```python
from build123d import *

# Parameters (mm, degrees)
F0_W           = 15.6
F0_H           = 5.8
F1_DEPTH       = 13.4
F2_W           = 1.5
F2_H           = 6.25
F3_DEPTH       = 1
F4_W           = 1.5
F4_H           = 6.25
F5_DEPTH       = 1
F6_W           = 13.6
F6_H           = 1
F7_DEPTH       = 1
F8_W           = 1.5
F8_H           = 6.3
F9_DEPTH       = 1
F10_W          = 1.3
F10_H          = 1.3
F11_DEPTH      = 13.401
F12_W          = 3.1
F12_H          = 4.1
F12_W_2        = 1.3
F12_H_2        = 1.3
F13_DEPTH      = 12.9
F15_DEPTH      = 3.75
F15_DEPTH_BACK = 3.75
F16_W          = 2.5
F16_H          = 8.7
F17_DEPTH      = 0.5


with BuildPart() as f1:
    # F0 (on Top) → F1 (new body)
    with BuildSketch(Plane.XY):
        Rectangle(F0_W, F0_H)
    extrude(amount=F1_DEPTH)

    # F2 (on face) → F3 (join)
    with BuildSketch(Plane.YZ.offset(7.8)):
        with Locations((3.65, 3.125)):
            Rectangle(F2_W, F2_H)
    extrude(amount=-F3_DEPTH)

    # F4 (on face) → F5 (join)
    with BuildSketch(Plane(origin=(-7.8, 0, 0), x_dir=(0, -1, 0), z_dir=(-1, 0, 0))):
        with Locations((-3.65, 3.125)):
            Rectangle(F4_W, F4_H)
    extrude(amount=-F5_DEPTH)

    # F6 (on face) → F7 (join)
    with BuildSketch(Plane.XZ.offset(2.9)):
        with Locations((0, 12.9)):
            Rectangle(F6_W, F6_H)
    extrude(amount=F7_DEPTH)

    # F8 (on face) → F9 (cut)
    with BuildSketch(Plane.XZ.offset(2.9)):
        with Locations((-6, 3.15)):
            Rectangle(F8_W, F8_H)
        with Locations((-2, 3.15)):
            Rectangle(F8_W, F8_H)
        with Locations((2, 3.15)):
            Rectangle(F8_W, F8_H)
        with Locations((6, 3.15)):
            Rectangle(F8_W, F8_H)
    extrude(amount=-F9_DEPTH, mode=Mode.SUBTRACT)

    # F10 (on Top) → F11 (cut, through all)
    with BuildSketch(Plane.XY):
        with Locations((5.94, 0.95)):
            Rectangle(F10_W, F10_H)
        with Locations((1.98, 0.95)):
            Rectangle(F10_W, F10_H)
        with Locations((-1.98, 0.95)):
            Rectangle(F10_W, F10_H)
        with Locations((-5.94, 0.95)):
            Rectangle(F10_W, F10_H)
    extrude(amount=F11_DEPTH, mode=Mode.SUBTRACT)

    # F12 (on face) → F13 (cut)
    with BuildSketch(Plane.XY.offset(13.4)):
        with Locations((-5.94, 0.1)):
            Rectangle(F12_W, F12_H)
        with Locations((-5.94, 0.95)):
            Rectangle(F12_W_2, F12_H_2, mode=Mode.SUBTRACT)
        with Locations((-1.98, 0.1)):
            Rectangle(F12_W, F12_H)
        with Locations((-1.98, 0.95)):
            Rectangle(F12_W_2, F12_H_2, mode=Mode.SUBTRACT)
        with Locations((1.98, 0.1)):
            Rectangle(F12_W, F12_H)
        with Locations((1.98, 0.95)):
            Rectangle(F12_W_2, F12_H_2, mode=Mode.SUBTRACT)
        with Locations((5.94, 0.1)):
            Rectangle(F12_W, F12_H)
        with Locations((5.94, 0.95)):
            Rectangle(F12_W_2, F12_H_2, mode=Mode.SUBTRACT)
    extrude(amount=-F13_DEPTH, mode=Mode.SUBTRACT)

    # F14 (on Right) → F15 (join, two sides)
    with BuildSketch(Plane.YZ) as f15_sk:
        with BuildLine():
            Line((3.5, 13.4), (2.9, 13.4))
            Line((2.9, 13.4), (2.9, 5.7))
            Line((2.9, 5.7), (3.5, 5.7))
            Line((3.5, 5.7), (3.5, 5.91))
            ThreePointArc((3.5, 5.91), (3.672807, 6.327193), (4.09, 6.5))
            Line((4.09, 6.5), (4.11, 6.5))
            ThreePointArc((4.11, 6.5), (4.527193, 6.327193), (4.7, 5.91))
            Line((4.7, 5.91), (4.7, 2.3))
            Line((4.7, 2.3), (6.1, 2.3))
            Line((6.1, 2.3), (6.1, 11))
            Line((6.1, 11), (7.132015, 11))
            Line((7.132015, 11), (7.132015, 12))
            Line((7.132015, 12), (4.7, 12))
            Line((4.7, 12), (4.7, 8.09))
            ThreePointArc((4.7, 8.09), (4.527193, 7.672807), (4.11, 7.5))
            Line((4.11, 7.5), (4.09, 7.5))
            ThreePointArc((4.09, 7.5), (3.672807, 7.672807), (3.5, 8.09))
            Line((3.5, 8.09), (3.5, 13.4))
        make_face()
    extrude(amount=F15_DEPTH)
    extrude(f15_sk.sketch, amount=-F15_DEPTH_BACK)

    # F16 (on face) → F17 (cut)
    with BuildSketch(Plane(origin=(0, 6.1, 0), x_dir=(-1, 0, 0), z_dir=(0, 1, 0))):
        with Locations((-2.5, 6.65)):
            Rectangle(F16_W, F16_H)
        with Locations((2.5, 6.65)):
            Rectangle(F16_W, F16_H)
    extrude(amount=-F17_DEPTH, mode=Mode.SUBTRACT)


solid = f1.part
```
Check sheet for the modelled part. Datum: model origin and axes. Units: mm. A direction names the side the tool comes from. Round coordinates to 2 decimals unless told otherwise and drop trailing zeros. Loops run counter-clockwise (first coordinate to the right, second up) from the corner with the lowest first, then second, coordinate; pieces in that order, holes last. Notation, with made-up numbers: (25.25, -13.5) -> (71.25, -13.5) arc R24 cw to (71.25, 15.5) -> close; hole circle Ø10 at (86.25, 68). An arc over 180 degrees is marked (long way). Write item = value, one per line. Start each with the question number.
1) Set-up check for faces 1 (the flat face through (-6.8, 4, 3)), 2 (the flat face through (-6, -2.4, 6.3)), 3 (the flat face through (-3.53, 0, 7)): record each of +Z, -Z, +X, -X, +Y, -Y from which the full face is reachable in a straight line by a thin tool's end or side.
2) Thickness scan on probe 1 along X at (y, z) = (-0.75, 11.75); probe 2 along Y at (x, z) = (2.5, 10); probe 3 along Y at (x, z) = (-0.5, 10). Record the ranges inside material, lowest first.
3) Sectioned sample at B-B, the plane x = -5.75. Record the cut outline in (y, z), plus the area to 3 significant figures.
4) Sectioned sample at C-C, the plane z = 7. Record the cut outline in (x, y), plus the area to 3 significant figures.
5) Release check for a two-part mould opening along X. For faces 4 (the flat face through (5.25, -2.4, 3.1)), 5 (the flat face through (0, -2.9, 7)) record: released by +X, released by -X, zero draft, split by the parting line, or undercut.
6) Sectioned sample at A-A, the plane z = 10.25. State how many separate pieces and enclosed holes the cut face has, plus the area to 3 significant figures.
7) Gauge pin test, flat ends, axial feed: pin 1 Ø0.6 at (y, z) = (6, 6) entering from +X; pin 2 Ø5 at (x, z) = (-3.5, 5.5) entering from -Y; pin 3 Ø6 at (x, z) = (1.5, 5) entering from +Y; pin 4 Ø1.5 at (y, z) = (-3, 10) entering from -X. Record the tip position at first contact, or that the pin passes through.
Results are:
q1.face_1 = +Z, -Z, +Y
q1.face_2 = -Z, -Y
q1.face_3 = +Z
q2.probe_1 = -7.8 to -7.49, -4.39 to -3.53, -0.43 to 0.43, 3.53 to 4.39, 7.49 to 7.8
q2.probe_2 = -2.9 to -1.95, 2.15 to 3.5, 4.7 to 5.6
q2.probe_3 = -2.9 to -1.95, 2.15 to 3.5, 4.7 to 6.1
q3.outline = (-3.9, 12.4) -> (-2.9, 12.4) -> (-2.9, 6.3) -> (-1.95, 6.3) -> (-1.95, 13.4) -> (-3.9, 13.4) -> close; (-1.9, 0) -> (0.3, 0) -> (0.3, 0.5) -> (-1.9, 0.5) -> close; (1.6, 0) -> (2.9, 0) -> (2.9, 13.4) -> (2.15, 13.4) -> (2.15, 0.5) -> (1.6, 0.5) -> close
q3.area = 19.2 mm^2
q4.outline = (-7.8, -2.9) -> (7.8, -2.9) -> (7.8, 2.9) -> (3.75, 2.9) -> (3.75, 5.6) -> (1.25, 5.6) -> (1.25, 6.1) -> (-1.25, 6.1) -> (-1.25, 5.6) -> (-3.75, 5.6) -> (-3.75, 2.9) -> (-7.8, 2.9) -> close; hole (-7.49, -1.95) -> (-4.39, -1.95) -> (-4.39, 2.15) -> (-7.49, 2.15) -> close; hole (-3.53, -1.95) -> (-0.43, -1.95) -> (-0.43, 2.15) -> (-3.53, 2.15) -> close; hole (0.43, -1.95) -> (3.53, -1.95) -> (3.53, 2.15) -> (0.43, 2.15) -> close; hole (4.39, -1.95) -> (7.49, -1.95) -> (7.49, 2.15) -> (4.39, 2.15) -> close
q4.area = 61.1 mm^2
q5.face_4 = undercut
q5.face_5 = zero draft
q6.separate_pieces = 2
q6.enclosed_holes = 4
q6.area = 52.1 mm^2
q7.pin_1 = 1.25
q7.pin_2 = -2.9
q7.pin_3 = 6.1
q7.pin_4 = -7.8
